Could you check a few things on this model? Use its own coordinates, in mm. A direction names the side the tool comes from. Round coordinates to 2 decimals unless told otherwise and drop trailing zeros. Order: outer loops, then holes, each group sorted by start corner. A loop starts at its lowest first (then second) coordinate and runs counter-clockwise, first axis right, second up. Notation, with made-up numbers: M 52,-40 L 105,-40 A15 cw 105,-13 Z; hole C 0,16.25 d4. An arc over 180 degrees is marked long. Write each question's results on one line, items separated by ' | '. Start each with the question number.
1. Please list where these lines run through material, in increasing order: L1, parallel to Y at x = 31.1, z = -6.65; L2, parallel to Y at x = 15, z = -6.5; L3, parallel to X at y = 13.5, z = -5.5.
2. Suppose I cut it at B-B on x = 5.1. Write out the boundary of the cut face in (y, z).
3. Suppose I cut it at A-A on y = 13.5. Write out the boundary of the cut face in (x, z).
4. Suppose I cut it at D-D on z = -6. Write out the boundary of the cut face in (x, y) (1 decimal), and give its area (3 significant figures).
5. I'm going to push flat-ended pins straight in: pin 1 (1.5 mm diameter, centred on x = 26, z = -1, fed in from +Y); pin 2 (2.5 mm diameter, centred on x = 23.5, z = -7, fed in from -Y); pin 3 (5 mm diameter, centred on x = 18.1, y = 13.5, fed in from -Z); pin 4 (1.7 mm diameter, centred on x = 25, y = 6, fed in from -Z). Where does each tip first touch, or does it pass through?
6. For faces 1 (the flat face through (31, 14, -5.62)), 2 (the cylindrical face through (23.13, 2.04, -4.32)), 3 (the cylindrical face through (35.75, 0.48, -5.23)), which set-ups out of +Z, -Z, +X, -X, +Y, -Y let a thin tool reach every point of the face, with its end or its side?
7. Suppose I cut it at C-C on x = 18.1. Write out the boundary of the cut face in (y, z).
Autodesk Inventor part; units mm, degrees
ref_plane "Work Plane1" through (23.0021, 0, -10.32) normal (1, 0, 0) x (0, 0, -1)
ref_plane "YZ Plane" through (0, 0, 0) normal (1, 0, 0) x (0, 1, 0)
ref_plane "XZ Plane" through (0, 0, 0) normal (0, 1, 0) x (-1, 0, 0)
sketch "Sketch1" plane through (0, 0, 0) normal (0, 0, 1) x (1, 0, 0)
  line L0 (0, 0) -> (36.2, 0)
  line L1 (36.2, 0) -> (36.2, 23)
  line L2 (36.2, 23) -> (0, 23)
  line L3 (0, 23) -> (0, 0)
  dimension "d0" = 36.2
  dimension "d1" = 23
extrude "Extrusion1" add sketch "Sketch1" against normal blind 10.32
sketch "Sketch2" plane through (0, 0, 0) normal (0, 0, 1) x (1, 0, 0)
  line L0 (0, 0) -> (36.2, 0)
  line L1 (36.2, 0) -> (36.2, 23)
  circle A0 centre (18.1, 13.5) radius 1.5
  dimension "d4" = 3
  dimension "d5" = 18.1
  dimension "d6" = 13.5
hole "Hole1" at (18.1, 13.5, 0) direction (0, 0, -1) diameter 3.2 end through all
sketch "Sketch3" plane through (0, 0, 0) normal (0, 0, 1) x (1, 0, 0)
  circle A0 centre (18.1, 13.5) radius 1.6
  line L0 (0, 0) -> (36.2, 0)
  line L1 (36.2, 0) -> (36.2, 23)
  line L2 (36.2, 23) -> (0, 23)
  line L3 (0, 23) -> (0, 0)
  line L4 (36.2, 21) -> (27.9042, 21)
  arc A1 (23.7521, 23) -> (27.9042, 21) centre (27.9042, 26.31) ccw
  arc A2 (13.9479, 23) -> (22.2521, 23) centre (18.1, 26.31) ccw
  line L5 (18.1, 21) -> (18.1, 0) construction
  dimension "d14" = 3.2
  dimension "d15" = 21
  dimension "d16" = 5.31
  dimension "d17" = 1.5
extrude "Extrusion2" cut sketch "Sketch3" against normal blind 10.32 contours L4 A1 L2 L1 | L2 A2
sketch "Sketch4" plane through (0, 0, -10.32) normal (0, 0, -1) x (-1, 0, 0)
  circle A0 centre (-18.1, 13.5) radius 1.6
  line L0 (-36.2, 21) -> (-36.2, 0)
  line L1 (0, 0) -> (0, 23)
  circle A1 centre (-31.1, 13.5) radius 3
  circle A2 centre (-5.1, 13.5) radius 3
  line L2 (-34.1, 13.5) -> (-36.2, 13.5)
  line L3 (-2.1, 13.5) -> (0, 13.5)
  point P0 (-35.15, 13.5)
  dimension "d21" = 6
  dimension "d20" = 26
extrude "Extrusion3" cut sketch "Sketch4" against normal blind 4.7 contours A1 | A2
sketch "Sketch6" plane through (0, 0, -10.32) normal (0, 0, -1) x (-1, 0, 0)
  line L0 (-22.2521, 23) -> (-23.7521, 23)
  line L1 (-36.2, 0) -> (0, 0)
  line L2 (-33.0021, 4.13) -> (-13.0021, 4.13)
  line L3 (-13.0021, 4.13) -> (-13.0021, 9.88)
  line L4 (-13.0021, 9.88) -> (-33.0021, 9.88)
  line L5 (-33.0021, 9.88) -> (-33.0021, 4.13)
  point P0 (-23.0021, 23)
  point P1 (-23.0021, 9.88)
  dimension "d27" = 5.75
  dimension "d28" = 20
  dimension "d29" = 4.13
extrude "Extrusion5" cut sketch "Sketch6" against normal blind 8.73
fillet "Fillet1" radius 1.5875 4 edges at (13.0021, 9.88, -5.955) (13.0021, 4.13, -5.955) (33.0021, 9.88, -5.955) (33.0021, 4.13, -5.955)
fillet "Fillet2" radius 1.5875 4 edges at (36.2, 21, -5.16) (36.2, 0, -5.16) (0, 0, -5.16) (0, 23, -5.16)
sketch "Sketch5" plane through (0, 0, 0) normal (0, -1, 0) x (1, 0, 0)
  line L0 (23.7521, 0) -> (22.2521, 0)
  circle A0 centre (23.0021, 0) radius 1 construction
  line L1 (36.2, -10.32) -> (0, -10.32)
  circle A1 centre (23.0021, -10.32) radius 1
  dimension "d24" = 2
extrude "Extrusion4" cut sketch "Sketch5" against normal through all
sketch "Sketch7" plane through (1.5875, 0, 0) normal (0, -1, 0) x (1, 0, 0)
  arc A0 (22.4146, -10.32) -> (20.4146, -10.32) centre (21.4146, -10.32) ccw
  circle A1 centre (21.4146, -10.32) radius 6
  point P0 (-1.5875, 0)
  dimension "d34" = 12
extrude "Extrusion6" cut sketch "Sketch7" against normal up to surface (4.13 mm away)
ref_plane "Work Plane1" through (23.0021, 0, -10.32) normal (1, 0, 0) x (0, 0, -1)
properties part number "hotend-holder-front"
Filled sheet:
1) L1: y = 0 to 4.13, 9.88 to 10.5, 16.5 to 21 | L2: y = 0 to 4.13, 9.88 to 22 | L3: x = 0 to 16.5, 19.7 to 36.2
2) outline: M 0,-10.32 L 10.5,-10.32 L 10.5,-5.62 L 16.5,-5.62 L 16.5,-10.32 L 23,-10.32 L 23,0 L 0,0 Z
3) outline: M 0,-10.32 L 2.1,-10.32 L 2.1,-5.62 L 8.1,-5.62 L 8.1,-10.32 L 16.5,-10.32 L 16.5,0 L 0,0 Z; M 19.7,-10.32 L 22,-10.32 A1 cw 24,-10.32 L 28.1,-10.32 L 28.1,-5.62 L 34.1,-5.62 L 34.1,-10.32 L 36.2,-10.32 L 36.2,0 L 19.7,0 Z
4) outline: M 0,1.6 A1.6 ccw 1.6,0 L 18.8,0 L 18.8,4.1 L 14.6,4.1 A1.6 cw 13,5.7 L 13,8.3 A1.6 cw 14.6,9.9 L 31.4,9.9 A1.6 cw 33,8.3 L 33,5.7 A1.6 cw 31.4,4.1 L 27.2,4.1 L 27.2,0 L 34.6,0 A1.6 ccw 36.2,1.6 L 36.2,19.4 A1.6 ccw 34.6,21 L 27.9,21 A5.3 cw 23.8,23 L 22.3,23 A5.3 cw 13.9,23 L 1.6,23 A1.6 ccw 0,21.4 Z; hole C 5.1,13.5 d6; hole C 18.1,13.5 d3.2; hole C 31.1,13.5 d6 | area: 585 mm^2
5) pin 1: stops at y = 21.71 | pin 2: stops at y = 9.88 | pin 3: stops at z = -10.32 | pin 4: stops at z = -1.59
6) face 1: -Z | face 2: -Z, -Y | face 3: +Z, -Z, +X, -Y
7) outline: M 0,-6.86 L 4.13,-6.86 L 4.13,-1.59 L 9.88,-1.59 L 9.88,-10.32 L 11.9,-10.32 L 11.9,0 L 0,0 Z; M 15.1,-10.32 L 21,-10.32 L 21,0 L 15.1,0 Z
